Geometry: final body of the model. Coordinates: model frame, mm. A direction names the side the tool comes from. Round coordinates to 2 decimals unless told otherwise and drop trailing zeros. Write each loop counter-clockwise with the first axis right and the second up, starting at its lowest first coordinate (ties: lowest second). Pieces come first, ordered by that corner, then holes. Notation, with made-up numbers: (54.25, -23) -> (98.25, -23) arc R26 ccw to (98.25, 5) -> close; hole circle Ø1 at (-27, 9). An arc over 180 degrees is marked (long way). One line per item, written item: value. Start each with the question number.
Autodesk Inventor part; units mm, degrees
ref_plane "YZ Plane" through (0, 0, 0) normal (1, 0, 0) x (0, 1, 0)
ref_plane "XZ Plane" through (0, 0, 0) normal (0, 1, 0) x (-1, 0, 0)
ref_plane "XY Plane" through (0, 0, 0) normal (0, 0, 1) x (1, 0, 0)
sketch "Sketch1" plane through (0, 0, 0) normal (0, 1, 0) x (-1, 0, 0)
  line L0 (4.6355, 50.8) -> (-4.6355, 50.8)
  line L1 (-4.6355, 50.8) -> (-4.6355, -50.8)
  line L2 (-4.6355, -50.8) -> (4.6355, -50.8)
  line L3 (4.6355, -50.8) -> (4.6355, 50.8)
  line L4 (4.6355, 50.8) -> (-4.6355, -50.8) construction
  line L5 (-4.6355, 50.8) -> (4.6355, -50.8) construction
  line L6 (4.6355, 50.8) -> (4.6355, 75.7051) construction
  line L7 (4.6355, -50.8) -> (4.6355, -91.0918) construction
  line L8 (-4.6355, 50.8) -> (4.6355, 60.071)
  line L9 (4.6355, 60.071) -> (-49.246, 113.9525)
  line L10 (-49.246, 113.9525) -> (-58.517, 104.6815)
  line L11 (-58.517, 104.6815) -> (-4.6355, 50.8)
  line L12 (-4.6355, 50.8) -> (8.4757, 50.8) construction
  line L13 (-4.6355, -50.8) -> (4.6355, -60.071)
  line L14 (4.6355, -60.071) -> (-49.246, -113.9525)
  line L15 (-49.246, -113.9525) -> (-58.517, -104.6815)
  line L16 (-58.517, -104.6815) -> (-4.6355, -50.8)
  line L17 (-4.6355, -50.8) -> (8.4757, -50.8) construction
  line L18 (4.6355, 60.071) -> (4.6355, 50.8)
  line L19 (4.6355, -50.8) -> (4.6355, -60.071)
  line L20 (4.6355, 50.8) -> (4.6355, 38.1)
  line L21 (4.6355, 41.021) -> (4.6355, 60.071)
  line L22 (4.6355, 31.75) -> (4.6355, 41.021)
  line L23 (48.5075, 0) -> (-17.0034, 0) construction
  line L24 (-58.517, -104.6815) -> (-58.517, 104.6815) construction
  line L25 (-49.246, -113.9525) -> (-58.517, -113.9525)
  line L26 (-58.517, -113.9525) -> (-58.517, -104.6815)
  line L27 (-58.517, -104.6815) -> (-94.077, -104.6815)
  line L28 (-94.077, -104.6815) -> (-94.077, -113.9525)
  line L29 (-94.077, -113.9525) -> (-58.517, -113.9525)
  line L30 (-58.517, 104.6815) -> (-94.077, 104.6815)
  line L31 (-94.077, 104.6815) -> (-94.077, 113.9525)
  line L32 (-94.077, 113.9525) -> (-49.246, 113.9525)
  line L33 (55.1879, -32) -> (4.6355, -32) construction
  line L34 (4.6355, -32) -> (4.6355, -60.071)
  line L35 (4.6355, 22.7291) -> (4.6355, 50.8)
  line L36 (33.8455, 32) -> (4.6355, 32) construction
  line L37 (4.6355, 32) -> (4.6355, 60.071)
  line L38 (4.6355, 27.3645) -> (33.8455, 27.3645) construction
  line L39 (33.8455, 27.3645) -> (33.8455, 36.6355)
  line L40 (33.8455, 36.6355) -> (4.6355, 36.6355) construction
  line L41 (4.6355, 36.6355) -> (4.6355, 27.3645)
  line L42 (4.6355, 27.3645) -> (33.8455, 36.6355) construction
  line L43 (33.8455, 27.3645) -> (4.6355, 36.6355) construction
  line L44 (4.6355, -32) -> (33.8455, -32) construction
  line L45 (4.6355, -36.6355) -> (33.8455, -36.6355) construction
  line L46 (33.8455, -36.6355) -> (33.8455, -27.3645)
  line L47 (33.8455, -27.3645) -> (4.6355, -27.3645) construction
  line L48 (4.6355, -27.3645) -> (4.6355, -36.6355)
  line L49 (4.6355, -36.6355) -> (33.8455, -27.3645) construction
  line L50 (33.8455, -36.6355) -> (4.6355, -27.3645) construction
  line L51 (33.8455, -32) -> (28.7655, -32) construction
  circle A0 centre (28.7655, -32) radius 1.85
  line L52 (33.8455, 32) -> (28.7655, 32) construction
  circle A1 centre (28.7655, 32) radius 1.85
  line L53 (33.8455, -36.6355) -> (4.6355, -47.2671)
  line L54 (33.8455, -36.6355) -> (64.9301, -36.6355) construction
  line L55 (33.8455, -27.3645) -> (4.6355, -16.7329)
  line L56 (33.8455, -27.3645) -> (64.9301, -27.3645) construction
  line L57 (33.8455, 27.3645) -> (4.6355, 16.7329)
  line L58 (33.8455, 27.3645) -> (64.9301, 27.3645) construction
  line L59 (33.8455, 36.6355) -> (4.6355, 47.2671)
  line L60 (33.8455, 36.6355) -> (64.9301, 36.6355) construction
  point P0 (0, 0)
  point P1 (33.8455, 45.6585)
  point P2 (33.8455, 45.6585)
  point P3 (33.8455, 45.6585)
  dimension "d0" = 9.271
  dimension "d1" = 101.6
  dimension "d2" = 45
  dimension "d3" = 76.2
  dimension "d4" = 45
  dimension "d5" = 76.2
  dimension "d8" = 12.7
  dimension "d12" = 35.56
  dimension "d17" = 35.56
  dimension "d28" = 9.271
  dimension "d29" = 50.5524
  dimension "d30" = 29.21
  dimension "d31" = 9.271
  dimension "d32" = 5.08
  dimension "d33" = 3.7
  dimension "d34" = 5.08
  dimension "d35" = 3.7
  dimension "d36" = 160
  dimension "d37" = 160
  dimension "d38" = 160
  dimension "d39" = 160
extrude "Extrusion4" add sketch "Sketch1" along normal blind 6.35
fillet "Fillet4" radius 3.175 6 edges at (49.246, 3.175, 113.9525) (49.246, 3.175, -113.9525) (-4.6355, 3.175, -47.2671) (-4.6355, 3.175, 16.7329) (-4.6355, 3.175, 47.2671) (-4.6355, 3.175, -16.7329)
fillet "Fillet5" radius 3.175 4 edges at (-33.8455, 3.175, 36.6355) (-33.8455, 3.175, -27.3645) (-33.8455, 3.175, 27.3645) (-33.8455, 3.175, -36.6355)
fillet "Fillet6" radius 3.175 2 edges at (4.6355, 3.175, 50.8) (4.6355, 3.175, -50.8)
properties part number "Arm"
(1) Set-up query: faces 5 (the face through (32.412, 3.131, 78.576)), 6 (the face through (-4.636, 3, 0)), 7 (the face through (-4.636, 3, 55)), 8 (the face through (2, 0, 1)), 9 (the face through (-19.416, 3.131, -41.888)). Return all of +Z, -Z, +X, -X, +Y, -Y with unobstructed straight access to the full face (end or side cutting, diameter ignored); none if empty.
(2) Section query D-D (z = 89). Output: boundary loops of the cut face in (x, y).
(3) Line query: probe 1 along Z at (x, y) = (71.5, 4.75); probe 2 along Z at (x, y) = (-7, 1); probe 3 along X at (y, z) = (6.25, -0.5). Output: solid intervals per line, ascending.
(4) Section query B-B (x = 67). Output: boundary loops of the cut face in (y, z).
(5) Pull-direction query (Z, two-part tool) for faces 1 (the face through (4.636, 3, 1)), 2 (the face through (-33.846, 3, 32)), 3 (the face through (21.47, 3.131, 86.176)), 4 (the face through (72, 3, -113.952)); classes: pulls with the +Z half, pulls with the -Z half, needs draft (parallel to the pull), parting line crosses it, or undercut.
(6) Section query C-C (x = 15.5). Output: boundary loops of the cut face in (y, z).
(7) Section query A-A (y = 1.75). Count the separate pieces of the cut face and the enclosed holes in it, and give its area (3 significant figures).
(8) Pin query (flat end, axial travel): pin 1 (2 mm diameter, centred on x = -28.77, z = -32, fed in from +Y); pin 2 (3 mm diameter, centred on y = 4.5, z = 75, fed in from -X); pin 3 (2 mm diameter, centred on x = 40, y = 5, fed in from -Z); pin 4 (3 mm diameter, centred on y = 3, z = 56.5, fed in from -X). Return the tip coordinate at first contact, or that it passes through.
Results list:
1. face 5: +X, +Y, -Y
1. face 6: -X, +Y, -Y
1. face 7: +Z, -X, +Y, -Y
1. face 8: +Z, -Z, +X, -X, -Y
1. face 9: -Z, -X, +Y, -Y
2. outline: (24.29, 0) -> (42.84, 0) -> (42.84, 6.35) -> (24.29, 6.35) -> close
3. probe 1: z = -113.95 to -104.68, 104.68 to 113.95
3. probe 2: z = -46.41 to -17.59, 17.59 to 46.41
3. probe 3: x = -4.64 to 4.64
4. outline: (0, -113.95) -> (6.35, -113.95) -> (6.35, -104.68) -> (0, -104.68) -> close; (0, 104.68) -> (6.35, 104.68) -> (6.35, 113.95) -> (0, 113.95) -> close
5. face 1: undercut
5. face 2: needs draft
5. face 3: pulls with the +Z half
5. face 4: pulls with the -Z half
6. outline: (0, -80.21) -> (6.35, -80.21) -> (6.35, -61.66) -> (0, -61.66) -> close; (0, 61.66) -> (6.35, 61.66) -> (6.35, 80.21) -> (0, 80.21) -> close
7. separate pieces: 1
7. enclosed holes: 2
7. area: 4,910 mm^2
8. pin 1: passes through
8. pin 2: stops at x = 8.79
8. pin 3: stops at z = -105.71
8. pin 4: stops at x = -4.64
